Geometry: see drawing. Coordinates: mm, zero at the bounding-box minimum. A direction names the side the tool comes from. Give positions to 0.01 mm unless a question says otherwise; leave off trailing zeros. Write each loop counter-clockwise with the first axis right and the second up, starting at its lowest first coordinate (ties: lowest second). Pieces come first, ordered by that corner, then holes. Notation, with made-up numbers: M -37.75,-34 L -32.75,-34 A26 ccw -32.75,-14 Z; hole C 35.25,66.25 d5. An arc over 180 degrees is marked long. Use CSV: the item, a comma, the result in double quotes. Start each with the question number.
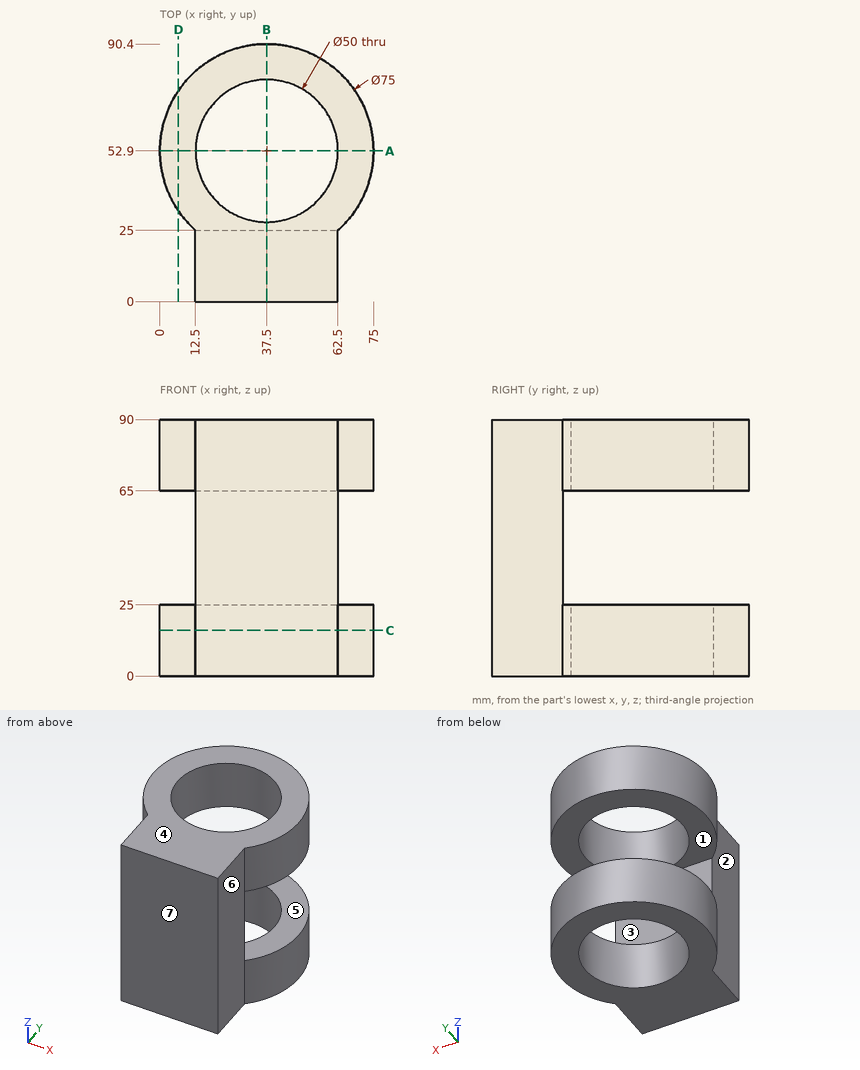
1. Section B-B on x = 37.5. Return loops of the section in (y, z), then the cut area to 3 significant figures.
2. Section D-D on x = 6.5. Return loops of the section in (y, z).
3. Section C-C on z = 16. Return loops of the section in (x, y).
4. Section A-A on y = 52.9. Return loops of the section in (x, z).
5. Access query for the marked faces 5, 6 and 7. Directions: +Z, -Z, +X, -X, +Y, -Y. A direction counts if a zero-diameter tool reaches every point of the face in a straight line with its end or side. Return the directions, or none.
6. Line query: probe 1 along Z at (x, y) = (9.5, 70); probe 2 along Y at (x, z) = (37.5, 12); probe 3 along X at (y, z) = (52, 8). Output: solid intervals per line, ascending.
7. Pull-direction query (Z, two-part tool) for the marked faces 1, 2, 3 and 4; classes: released by +Z, released by -Z, zero draft, split by the parting line, or undercut.
8. First-contact query: pin 1 (20 mm diameter, centred on x = 44.5, z = 39, fed in from +Y); pin 2 (1 mm diameter, centred on x = 42, z = 23.5, fed in from +Y); pin 3 (20 mm diameter, centred on y = 16.5, z = 52, fed in from -X); pin 4 (19.5 mm diameter, centred on x = 35, y = 65.5, fed in from +Z) (3 decimals). Flat tips, straight axial feed; report the tip coordinate or a pass-through.
Resolved:
1,outline,"M 0,0 L 27.9,0 L 27.9,25 L 25,25 L 25,65 L 27.9,65 L 27.9,90 L 0,90 Z; M 77.9,0 L 90.4,0 L 90.4,25 L 77.9,25 Z; M 77.9,65 L 90.4,65 L 90.4,90 L 77.9,90 Z"
1,area,"3,020 mm2"
2,outline,"M 31.8,0 L 74,0 L 74,25 L 31.8,25 Z; M 31.8,65 L 74,65 L 74,90 L 31.8,90 Z"
3,outline,"M 12.5,0 L 62.5,0 L 62.5,24.95 A37.5 ccw long 12.5,24.95 Z; hole C 37.5,52.9 d50"
4,outline,"M 0,0 L 12.5,0 L 12.5,25 L 0,25 Z; M 0,65 L 12.5,65 L 12.5,90 L 0,90 Z; M 62.5,0 L 75,0 L 75,25 L 62.5,25 Z; M 62.5,65 L 75,65 L 75,90 L 62.5,90 Z"
5,face 5,"+X, -X, +Y"
5,face 6,"+Z, -Z, +X, -Y"
5,face 7,"+Z, -Z, +X, -X, -Y"
6,probe 1,"z = 0 to 25, 65 to 90"
6,probe 2,"y = 0 to 27.9, 77.9 to 90.4"
6,probe 3,"x = 0.01 to 12.52, 62.48 to 74.99"
7,face 1,"undercut"
7,face 2,"zero draft"
7,face 3,"undercut"
7,face 4,"released by +Z"
8,pin 1,"stops at y = 25"
8,pin 2,"stops at y = 90.19"
8,pin 3,"stops at x = 12.5"
8,pin 4,"passes through"
